from build123d import *

# Parameters (mm, degrees)
F0_R     = 5
F1_DEPTH = 3
F2_W     = 3
F2_H     = 80
F3_DEPTH = 25
F2_W_2   = 22
F4_DEPTH = 3
F5_R     = 2
F6_DEPTH = 150
F7_R     = 2
F8_DEPTH = 25


with BuildPart() as f1:
    # F0 (on Front) → F1 (new body)
    with BuildSketch(Plane.XZ):
        with BuildLine():
            ThreePointArc((0, 10), (2.928932, 2.928932), (10, 0))
            Line((10, 0), (140, 0))
            ThreePointArc((140, 0), (147.071068, 2.928932), (150, 10))
            Line((150, 10), (150, 140))
            ThreePointArc((150, 140), (147.071068, 147.071068), (140, 150))
            Line((140, 150), (10, 150))
            ThreePointArc((10, 150), (2.928932, 147.071068), (0, 140))
            Line((0, 140), (0, 10))
        make_face()
        with Locations((83, 75)):
            Circle(F0_R, mode=Mode.SUBTRACT)
    extrude(amount=F1_DEPTH)

    # F2 (on face) → F3 (join)
    with BuildSketch(Plane(origin=(0, 0, 0), x_dir=(-1, 0, 0), z_dir=(0, 1, 0))):
        with Locations((-118.5, 75)):
            Rectangle(F2_W, F2_H)
        with Locations((-33.5, 75)):
            Rectangle(F2_W, F2_H)
    extrude(amount=F3_DEPTH)

    # F2 (on face) → F4 (join)
    with BuildSketch(Plane(origin=(0, 0, 0), x_dir=(-1, 0, 0), z_dir=(0, 1, 0))):
        with Locations((-106, 75)):
            Rectangle(F2_W_2, F2_H)
        with Locations((-118.5, 75)):
            Rectangle(F2_W, F2_H)
        with Locations((-46, 75)):
            Rectangle(F2_W_2, F2_H)
        with Locations((-33.5, 75)):
            Rectangle(F2_W, F2_H)
    extrude(amount=F4_DEPTH)

    # F5 (on face) → F6 (cut)
    with BuildSketch(Plane.YZ.offset(120)):
        with Locations((15, 105)):
            Circle(F5_R)
        with Locations((15, 45)):
            Circle(F5_R)
    extrude(amount=-F6_DEPTH, mode=Mode.SUBTRACT)

    # F7 (on face) → F8 (cut)
    with BuildSketch(Plane(origin=(0, 3, 0), x_dir=(-1, 0, 0), z_dir=(0, 1, 0))):
        with Locations((-46, 45)):
            Circle(F7_R)
        with Locations((-46, 105)):
            Circle(F7_R)
        with Locations((-106, 45)):
            Circle(F7_R)
        with Locations((-106, 105)):
            Circle(F7_R)
    extrude(amount=-F8_DEPTH, mode=Mode.SUBTRACT)


solid = f1.part
Design review of the part built by this model. Coordinates are the model's own, in mm. A direction names the side the tool comes from. Give positions to 0.01 mm unless a question says otherwise; leave off trailing zeros. Loops run counter-clockwise (first coordinate to the right, second up) from the corner with the lowest first, then second, coordinate; pieces in that order, holes last. Notation, with made-up numbers: M 5,39 L 63,39 A31 ccw 63,77 Z; hole C -6,-26 d4. An arc over 180 degrees is marked long. One line per question, with ' | ' between items. Start each with the question number.
1. Add section A-A (z = 75). Write out the cut boundary in (x, y), plus the area to 3 significant figures.
2. Add section B-B (y = 9.5). Write out the cut boundary in (x, z).
3. Insertion check: P1, Ø2.5, axis at y = 1.5, z = 91.5, coming from the -X side; P2, Ø13, axis at x = 83, z = 75, coming from the +Y side; P3, Ø11, axis at x = 43.5, z = 63.5, coming from the +Y side; P4, Ø2.5, axis at y = 15, z = 105, coming from the -X side. Each pin has a flat end and moves straight along its axis. Give the tip position at first contact, or say it passes through.
4. Add section C-C (x = 46). Write out the cut boundary in (y, z), plus the area to 3 significant figures.
5. Add section D-D (x = 83). Write out the cut boundary in (y, z).
6. To check wall thickness, follow L1, parallel to Z at x = 33.5, y = 15; L2, parallel to Z at x = 106, y = -0.25; L3, parallel to X at y = 24.25, z = 85. State the ranges of each line that lie inside material, in increasing order.
7. For faces 1 (the face through (112, 2, 115)), 2 (the face through (120, 12, 74)), 3 (the face through (106, 3, 76)), 4 (the face through (34, 15, 107)), list the 3-axis set-ups (+Z, -Z, +X, -X, +Y, -Y) from which the entire face can be reached by the end or side of a thin tool; tool diameter is ignored.
8. The part is to be moulded in two halves that separate along X. For faces 5 (the face through (35, 14, 74)), 6 (the face through (46, 0, 107)), 7 (the face through (3.01, -1.48, 147.15)), 8 (the face through (34, 7, 115)), say which applies: released by +X, released by -X, zero draft, split by the parting line, or undercut.
Worked out:
1) outline: M 0,-3 L 78,-3 L 78,0 L 57,0 L 57,3 L 35,3 L 35,25 L 32,25 L 32,0 L 0,0 Z; M 88,-3 L 150,-3 L 150,0 L 120,0 L 120,25 L 117,25 L 117,3 L 95,3 L 95,0 L 88,0 Z | area: 702 mm²
2) outline: M 32,35 L 35,35 L 35,115 L 32,115 Z; M 117,35 L 120,35 L 120,115 L 117,115 Z
3) P1: stops at x = 32 | P2: stops at y = 0 | P3: stops at y = 3 | P4: passes through
4) outline: M -3,0 L 0,0 L 0,35 L 3,35 L 3,43 L -3,43 Z; M -3,47 L 3,47 L 3,103 L -3,103 Z; M -3,107 L 3,107 L 3,115 L 0,115 L 0,150 L -3,150 Z | area: 642 mm²
5) outline: M -3,0 L 0,0 L 0,70 L -3,70 Z; M -3,80 L 0,80 L 0,150 L -3,150 Z
6) L1: z = 35 to 43, 47 to 103, 107 to 115 | L2: z = 0 to 43, 47 to 103, 107 to 150 | L3: x = 32 to 35, 117 to 120
7) face 1: +Z, +X, -X, +Y | face 2: +Z, -Z, +X, +Y | face 3: +Z, -Z, +Y | face 4: +X, -X
8) face 5: undercut | face 6: undercut | face 7: released by -X | face 8: zero draft
